from build123d import *

# Parameters (mm, degrees)
SKETCH2_R           = 2.5
BOSS_EXTRUDE1_DEPTH = 10
BOSS_EXTRUDE2_DEPTH = 10


with BuildPart() as part:
    # Sketch2 → Boss-Extrude1 (new body)
    with BuildSketch(Plane(origin=(0, 0, 0), x_dir=(1, 0, 0), z_dir=(0, 1, 0))):
        with BuildLine():
            Line((-33.226342232, -9.981880582), (-27.883647244, -9.981880582))
            Line((-27.883647244, -9.981880582), (-27.883647244, 29.925281779))
            ThreePointArc((-27.883647244, 29.925281779), (-27.956490633, 31.630693582), (-28.174490185, 33.323682587))
            ThreePointArc((-28.174490185, 33.323682587), (-5.126582747, 60.257622762), (25.614975975, 42.605434852))
            ThreePointArc((25.614975975, 42.605434852), (34.529334698, 29.401291822), (48.478573237, 21.70493367))
            ThreePointArc((48.478573237, 21.70493367), (55.54506633, 25.728573237), (51.521426763, 32.79506633))
            ThreePointArc((51.521426763, 32.79506633), (43.044695487, 37.228328186), (37.173927096, 44.781000713))
            Line((37.173927096, 44.781000713), (29.544453309, 60.710630122))
            ThreePointArc((29.544453309, 60.710630122), (3.323171133, 73.595527675), (-24.801894282, 65.686234454))
            add(Edge.make_bspline(
                [(-36.866842145, 26.021473673), (-43.224794525, 50.957582374), (-24.801894282, 65.686234454)],
                knots=[0, 0, 0, 1, 1, 1], degree=2))
            Line((-36.866842145, 26.021473673), (-35.540312543, 23.509134839))
            ThreePointArc((-35.540312543, 23.509134839), (-33.813452265, 18.981182225), (-33.226342232, 14.170807697))
            Line((-33.226342232, 14.170807697), (-33.226342232, -9.981880582))
        make_face()
        with Locations(Location((0, 67.25, 0), (0, 0, 270))):
            Circle(SKETCH2_R, mode=Mode.SUBTRACT)
        with Locations(Location((50, 27.25, 0), (0, 0, 270))):
            Circle(SKETCH2_R, mode=Mode.SUBTRACT)
    extrude(amount=BOSS_EXTRUDE1_DEPTH)

    # Sketch1 → Boss-Extrude2 (add)
    with BuildSketch(Plane(origin=(0, 0, 0), x_dir=(1, 0, 0), z_dir=(0, 1, 0))):
        Polygon((-26.25, 10.75), (-15, 10.75), (-15, 0), (-23.984756923, -9), (-26.25, -9), (-26.25, -0.114272299), (-29.438415679, -2.555067389), (-29.438415679, 11.073293435), (-26.25, 9.911985917), align=None)
    extrude(amount=BOSS_EXTRUDE2_DEPTH)


solid = part.part
Input: part model. Units: mm. Frame: model coordinates. A direction names the side the tool comes from. Coordinates: 2 decimals unless noted, no trailing zeros. Order: outer loops, then holes, each group sorted by start corner. A loop starts at its lowest first (then second) coordinate and runs counter-clockwise, first axis right, second up. Notation, with made-up numbers: M 59,54 L 68,54 A36 ccw 68,89 Z; hole C 67.5,-33 d11. An arc over 180 degrees is marked long. Answer as CSV lines item,"result".
1. Section C-C (y = 1.25). State how many separate pieces and enclosed holes the cut face has, then the cut area to 3 significant figures.
Reported:
separate pieces,"1"
enclosed holes,"2"
area,"1,980 mm2"
2. Section A-A (z = -67.25). Return the cut outline in (x, y).
Reported:
outline,"M -22.55,0 L -2.5,0 L -2.5,10 L -22.55,10 Z; M 2.5,0 L 21.74,0 L 21.74,10 L 2.5,10 Z"
3. Access query for faces 4 (the flat face through (-21, 5, -10.75)), 5 (the cylindrical face through (34.364, 4.93, -29.554)), 6 (the cylindrical face through (-27.954, 4.93, -31.607)). Directions: +Z, -Z, +X, -X, +Y, -Y. A direction counts if a zero-diameter tool reaches every point of the face in a straight line with its end or side. Return the directions, or none.
Reported:
face 4,"+X, +Y, -Y"
face 5,"+Z, +Y, -Y"
face 6,"+Y, -Y"
4. Section D-D (x = 21). Return the cut outline in (y, z), then the cut area to 3 significant figures.
Reported:
outline,"M 0,-67.71 L 10,-67.71 L 10,-50.59 L 0,-50.59 Z"
area,"171 mm2"
5. First-contact query: P1, Ø5, axis at y = 2.5, z = -4, coming from the +X side; P2, Ø4, axis at y = 1, z = -4.5, coming from the -X side; P3, Ø3, axis at x = -19.5, y = 4.5, coming from the -Z side. Flat tips, straight axial feed; report the tip coordinate or a pass-through.
Reported:
P1,"x = -15"
P2,"x = -33.23"
P3,"z = -69.78"
6. Pull-direction query (X, two-part tool) for faces 1 (the flat face through (-33.226, 5, -2)), 2 (the cylindrical face through (-5.66, 4.93, -60.16)), 3 (the flat face through (-25, 5, 9)); classes: released by +X, released by -X, zero draft, split by the parting line, or undercut.
Reported:
face 1,"released by -X"
face 2,"undercut"
face 3,"zero draft"
7. Material intervals for line 1 (X direction, y = 7, z = -27.25); line 2 (X direction, y = 3.5, z = -28); line 3 (X direction, y = 3.5, z = -41), sorted ascending. Write a range as from..to.
Reported:
line 1,"-37.17..-27.88, 37.13..47.5, 52.5..55.75"
line 2,"-37.34..-27.88, 36.16..47.62, 52.38..55.7"
line 3,"-38.39..-26.97, 26.26..39.47"
8. Section B-B (x = 50). Return the cut outline in (y, z).
Reported:
outline,"M 0,-33.27 L 10,-33.27 L 10,-29.75 L 0,-29.75 Z; M 0,-24.75 L 10,-24.75 L 10,-21.5 L 0,-21.5 Z"
